from build123d import *

# Parameters (mm, degrees)
SKETCH1_W           = 12
SKETCH1_H           = 10
BOSS_EXTRUDE1_DEPTH = 15
CUT_EXTRUDE1_DEPTH  = 17.911534525
SKETCH3_R           = 2.5
BOSS_EXTRUDE2_DEPTH = 1.25
SKETCH4_W           = 1.25
SKETCH4_H           = 1.5
SKETCH4_R           = 0.125
BOSS_EXTRUDE3_DEPTH = 0.25
FILLET2_R           = 0.5
SKETCH5_W           = 12
SKETCH5_H           = 10
BOSS_EXTRUDE4_DEPTH = 9
FILLET1_R           = 0.5
SKETCH6_R           = 1.5
BOSS_EXTRUDE5_DEPTH = 9.5
CHAMFER1_SIZE       = 0.5
CUT_EXTRUDE2_START  = -6
CUT_EXTRUDE2_DEPTH  = 6


with BuildPart() as part:
    # Sketch1 → Boss-Extrude1 (new body)
    with BuildSketch(Plane.XY):
        Rectangle(SKETCH1_W, SKETCH1_H)
    extrude(amount=BOSS_EXTRUDE1_DEPTH)

    # Sketch2 → Cut-Extrude1 (cut, through all)
    with BuildSketch(Plane.XY.offset(15)):
        with BuildLine():
            ThreePointArc((-6, 0), (-5.267141914, 2.853178053), (-3.25, 5))
            Line((-3.25, 5), (-6, 5))
            Line((-6, 5), (-6, 0))
        make_face()
        with BuildLine():
            ThreePointArc((-3.25, -5), (-5.267141914, -2.853178053), (-6, 0))
            Line((-6, 0), (-6, -5))
            Line((-6, -5), (-3.25, -5))
        make_face()
    cut_extrude1 = extrude(amount=-CUT_EXTRUDE1_DEPTH, mode=Mode.SUBTRACT)

    # Mirror1: Cut-Extrude1 across plane
    add(cut_extrude1.mirror(Plane(origin=(0, 0, 0), x_dir=(0, 0, 1), z_dir=(1, 0, 0))), mode=Mode.SUBTRACT)

    # Sketch3 → Boss-Extrude2 (add)
    with BuildSketch(Plane(origin=(0, 0, 0), x_dir=(-1, 0, 0), z_dir=(0, 0, -1))):
        Circle(SKETCH3_R)
    extrude(amount=BOSS_EXTRUDE2_DEPTH)

    # Sketch4 → Boss-Extrude3 (add)
    with BuildSketch(Plane(origin=(4, 0, 0), x_dir=(0, 0, -1), z_dir=(1, 0, 0))):
        with Locations((0.625, 0)):
            Rectangle(SKETCH4_W, SKETCH4_H)
        with Locations((0.625, 0)):
            Circle(SKETCH4_R, mode=Mode.SUBTRACT)
    boss_extrude3 = extrude(amount=-BOSS_EXTRUDE3_DEPTH)

    # Mirror2: Boss-Extrude3 across plane
    add(boss_extrude3.mirror(Plane(origin=(0, 0, 0), x_dir=(0, 0, 1), z_dir=(1, 0, 0))))

    # Fillet2
    fillet2_edges = [part.edges().sort_by_distance(p)[0] for p in [
        (-6, 0, 15),
        (0, -5, 15),
        (0, 5, 15),
        (6, 0, 15),
    ]]
    fillet(fillet2_edges, radius=FILLET2_R)

    # Sketch5 → Boss-Extrude4 (add)
    with BuildSketch(Plane.XY.offset(15)):
        Rectangle(SKETCH5_W, SKETCH5_H)
    extrude(amount=BOSS_EXTRUDE4_DEPTH)

    # Fillet1
    fillet1_edges = [part.edges().sort_by_distance(p)[0] for p in [
        (6, 5, 19.5),
        (-6, 5, 19.5),
        (-6, -5, 19.5),
        (6, -5, 19.5),
    ]]
    fillet(fillet1_edges, radius=FILLET1_R)

    # Sketch6 → Boss-Extrude5 (add)
    with BuildSketch(Plane.XY.offset(24)):
        Circle(SKETCH6_R)
    extrude(amount=BOSS_EXTRUDE5_DEPTH)

    # Chamfer1
    chamfer1_edges = [part.edges().sort_by_distance(p)[0] for p in [
        (-1.5, 0, 24),
    ]]
    chamfer(chamfer1_edges, length=CHAMFER1_SIZE)

    # Sketch7 → Cut-Extrude2 (cut)
    with BuildSketch(Plane.XY.offset(33.5).offset(CUT_EXTRUDE2_START)):
        with BuildLine():
            Line((-1.118033989, -1), (1.118033989, -1))
            ThreePointArc((1.118033989, -1), (0, -1.5), (-1.118033989, -1))
        make_face()
    extrude(amount=CUT_EXTRUDE2_DEPTH, mode=Mode.SUBTRACT)


solid = part.part
Source: CAD feature listing. Evaluate the final solid. Frame: model axes, mm. A direction names the side the tool comes from. Coordinates: 2 decimals unless noted, no trailing zeros. Order: outer loops, then holes, each group sorted by start corner. A loop starts at its lowest first (then second) coordinate and runs counter-clockwise, first axis right, second up.
Item 1: First-contact query: P1, Ø6, axis at y = -3, z = 3, coming from the +X side; P2, Ø1.4, axis at y = -0.5, z = -1, coming from the +X side; P3, Ø0.7, axis at x = -0.5, z = 31, coming from the -Y side; P4, Ø0.6, axis at y = 0, z = -0.5, coming from the -X side. Flat tips, straight axial feed; report the tip coordinate or a pass-through.
Output values:
P1: stops at x = 6
P2: stops at x = 4
P3: stops at y = -1
P4: stops at x = -4
Item 2: Material intervals for line 1 (Z direction, x = 2, y = 2.5); line 2 (X direction, y = 0.25, z = 12); line 3 (X direction, y = 4, z = 1), sorted ascending.
Output values:
line 1: z = 0 to 24
line 2: x = -5.99 to 5.99
line 3: x = -4.44 to 4.44
Item 3: Cut plane A-A (x = 0). Return loops of the section in (y, z), plus the area to 3 significant figures.
Output values:
outline: (-5, 0) - (-2.5, 0) - (-2.5, -1.25) - (2.5, -1.25) - (2.5, 0) - (5, 0) - (5, 14.5) arc R0.5 ccw to (4.5, 15) - (5, 15) - (5, 24) - (2, 24) - (1.5, 24.5) - (1.5, 33.5) - (-1, 33.5) - (-1, 27.5) - (-1.5, 27.5) - (-1.5, 24.5) - (-2, 24) - (-5, 24) - (-5, 15) - (-4.5, 15) arc R0.5 ccw to (-5, 14.5) - close
area: 272 mm2
Item 4: Cut plane C-C (z = 28). Return loops of the section in (x, y), plus the area to 3 significant figures.
Output values:
outline: (-1.12, -1) - (1.12, -1) arc R1.5 ccw (long way) to start
area: 6.29 mm2
Item 5: Cut plane B-B (z = 6). Return loops of the section in (x, y), plus the area to 3 significant figures.
Output values:
outline: (-3.25, -5) - (3.25, -5) arc R5.92 ccw to (3.25, 5) - (-3.25, 5) arc R5.92 ccw to start
area: 104 mm2
Item 6: Set-up query: faces 1 (the face through (3.75, 0, -1)), 2 (the face through (-0.195, 1.487, 28.937)), 3 (the face through (0, -1, 30)). Return all of +Z, -Z, +X, -X, +Y, -Y with unobstructed straight access to the full face (end or side cutting, diameter ignored); none if empty.
Output values:
face 1: -Z, +Y, -Y
face 2: +Z
face 3: +Z, +X, -X, -Y
